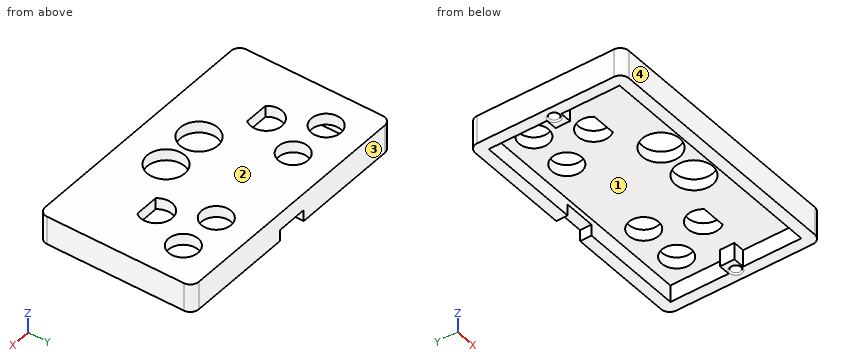
from build123d import *

# Parameters (mm, degrees)
SKETCH_W        = 46
SKETCH_H        = 27
PAD_DEPTH       = 3
SKETCH001_W     = 46
SKETCH001_H     = 27
SKETCH001_R     = 2.6
SKETCH001_R_2   = 3.3
PAD001_DEPTH    = 2
SKETCH002_W     = 5.5
SKETCH002_H     = 2
POCKET_DEPTH    = 2
SKETCH003_R     = 0.875
POCKET001_DEPTH = 2.5
FILLET_R        = 1.5
FILLET001_R     = 0.25


with BuildPart() as part:
    # Sketch → Pad (new body)
    with BuildSketch(Plane.XY):
        Rectangle(SKETCH_W, SKETCH_H)
        Polygon((-21, 11.5), (21, 11.5), (21, 1.27), (19, 1.27), (19, -1.27), (21, -1.27), (21, -11.5), (-21, -11.5), (-21, -1.27), (-19, -1.27), (-19, 1.27), (-21, 1.27), align=None, mode=Mode.SUBTRACT)
    extrude(amount=PAD_DEPTH)

    # Sketch001 (on Face18 of Pad) → Pad001 (join)
    with BuildSketch(Plane.XY.offset(3)):
        Rectangle(SKETCH001_W, SKETCH001_H)
        with Locations((-16.51, 6.985)):
            Circle(SKETCH001_R, mode=Mode.SUBTRACT)
        with Locations((-8.89, 6.985)):
            Circle(SKETCH001_R, mode=Mode.SUBTRACT)
        with Locations((8.89, 6.985)):
            Circle(SKETCH001_R, mode=Mode.SUBTRACT)
        with Locations((16.51, 6.985)):
            Circle(SKETCH001_R, mode=Mode.SUBTRACT)
        with Locations((-3.81, -5.715)):
            Circle(SKETCH001_R_2, mode=Mode.SUBTRACT)
        with Locations((3.81, -5.715)):
            Circle(SKETCH001_R_2, mode=Mode.SUBTRACT)
        with BuildLine():
            ThreePointArc((-10.575, -2.38053), (-12.7, 2.115), (-14.825, -2.38053))
            Line((-14.825, -2.38053), (-10.575, -2.38053))
        make_face(mode=Mode.SUBTRACT)
        with BuildLine():
            ThreePointArc((14.825, -2.38053), (12.7, 2.115), (10.575, -2.38053))
            Line((10.575, -2.38053), (14.825, -2.38053))
        make_face(mode=Mode.SUBTRACT)
    extrude(amount=PAD001_DEPTH)

    # Sketch002 (on Face4 of Pad001) → Pocket (cut)
    with BuildSketch(Plane(origin=(0, 0, 0), x_dir=(1, 0, 0), z_dir=(0, 0, -1))):
        with Locations((0, -12.5)):
            Rectangle(SKETCH002_W, SKETCH002_H)
    extrude(amount=-POCKET_DEPTH, mode=Mode.SUBTRACT)

    # Sketch003 (on Face2 of Pocket) → Pocket001 (cut)
    with BuildSketch(Plane(origin=(0, 0, 0), x_dir=(1, 0, 0), z_dir=(0, 0, -1))):
        with Locations((21, 0)):
            Circle(SKETCH003_R)
        with Locations((-21, 0)):
            Circle(SKETCH003_R)
    extrude(amount=-POCKET001_DEPTH, mode=Mode.SUBTRACT)

    # Fillet
    fillet_edges = [part.edges().sort_by_distance(p)[0] for p in [
        (-23, -13.5, 1.5),
        (23, -13.5, 1.5),
        (-23, 13.5, 1.5),
        (23, 13.5, 1.5),
    ]]
    fillet(fillet_edges, radius=FILLET_R)

    # Fillet001
    fillet001_edges = [part.edges().sort_by_distance(p)[0] for p in [
        (-21.875, 0, 0),
        (20.125, 0, 0),
    ]]
    fillet(fillet001_edges, radius=FILLET001_R)


solid = part.part
The model under review builds one solid part; all positions refer to its coordinate system, in mm. Face numbers are marked on the shaded views. Round coordinates to 2 decimals unless told otherwise and drop trailing zeros. Order: outer loops, then holes, each group sorted by start corner. A loop starts at its lowest first (then second) coordinate and runs counter-clockwise, first axis right, second up. Notation, with made-up numbers: (-30.75, 54.25) -> (27.25, 54.25) arc R20 ccw to (27.25, 85.25) -> close; hole circle Ø6 at (9.25, -16). An arc over 180 degrees is marked (long way). Return JSON: item names as keys, results as strings.
1. The part is to be moulded in two halves that separate along Y. For the marked faces 1, 2, 3 and 4, say which applies: +Y half, -Y half, draft (parallel to the pull), parting line (faces both ways), or undercut.
Answer block:
{"face 1": "undercut", "face 2": "draft", "face 3": "+Y half", "face 4": "-Y half"}
2. Take a section at D-D (y = -3). Write out the cut boundary in (x, z).
Answer block:
{"outline": "(-23, 0) -> (-21, 0) -> (-21, 3) -> (-5.69, 3) -> (-5.69, 5) -> (-23, 5) -> close; (-1.93, 3) -> (1.93, 3) -> (1.93, 5) -> (-1.93, 5) -> close; (5.69, 3) -> (21, 3) -> (21, 0) -> (23, 0) -> (23, 5) -> (5.69, 5) -> close"}
3. Insertion check: P1, Ø3, axis at x = -8.89, y = 6.985, coming from the +Z side; P2, Ø4.5, axis at x = 12.7, y = -0.635, coming from the -Z side. Each pin has a flat end and moves straight along its axis. Give the tip position at first contact, or say it passes through.
Answer block:
{"P1": "passes through", "P2": "stops at z = 3"}
4. For L1, parallel to X at y = -5.5, z = 4.75; L2, parallel to Y at x = -3, z = 2.1; L3, parallel to Y at x = 4, z = 3.75, list the stretches that pass through material, from the lowest coordinate up. Write a range as [from, to].
Answer block:
{"L1": "x = [-23, -7.1], [-0.52, 0.52], [7.1, 23]", "L2": "y = [-13.5, -11.5], [11.5, 13.5]", "L3": "y = [-13.5, -9.01], [-2.42, 13.5]"}
5. Take a section at B-B (z = 1.55). Write out the cut boundary in (x, y) (3 decimals).
Answer block:
{"outline": "(-23, -12) arc R1.5 ccw to (-21.5, -13.5) -> (21.5, -13.5) arc R1.5 ccw to (23, -12) -> (23, 12) arc R1.5 ccw to (21.5, 13.5) -> (2.75, 13.5) -> (2.75, 11.5) -> (21, 11.5) -> (21, 1.27) -> (19, 1.27) -> (19, -1.27) -> (21, -1.27) -> (21, -11.5) -> (-21, -11.5) -> (-21, -1.27) -> (-19, -1.27) -> (-19, 1.27) -> (-21, 1.27) -> (-21, 11.5) -> (-2.75, 11.5) -> (-2.75, 13.5) -> (-21.5, 13.5) arc R1.5 ccw to (-23, 12) -> close; hole circle Ø1.75 at (-21, 0); hole circle Ø1.75 at (21, 0)"}
6. Take a section at A-A (x = 3.81). Write out the cut boundary in (y, z) (3 decimals), then the cut area to 3 significant figures.
Answer block:
{"outline": "(-13.5, 0) -> (-11.5, 0) -> (-11.5, 3) -> (-9.015, 3) -> (-9.015, 5) -> (-13.5, 5) -> close; (-2.415, 3) -> (11.5, 3) -> (11.5, 0) -> (13.5, 0) -> (13.5, 5) -> (-2.415, 5) -> close", "area": "52.8 mm²"}
7. Take a section at C-C (y = -10.25). Write out the cut boundary in (x, z).
Answer block:
{"outline": "(-23, 0) -> (-21, 0) -> (-21, 3) -> (21, 3) -> (21, 0) -> (23, 0) -> (23, 5) -> (-23, 5) -> close"}
